CAD build for the part. Positions are in the model's coordinates, mm. Round coordinates to 2 decimals unless told otherwise and drop trailing zeros. Loops run counter-clockwise (first coordinate to the right, second up) from the corner with the lowest first, then second, coordinate; pieces in that order, holes last. Notation, with made-up numbers: M -0.5,20.25 L 42.5,20.25 A5 ccw 42.5,26.25 Z; hole C 84.25,-20.75 d1. An arc over 180 degrees is marked long. Use a Markdown table: item, result. Add a question column.
(1) Band-saw the part on D-D, the plane x = -10. Write the cut outline in (y, z), and give its area (3 significant figures).
(2) Band-saw the part on C-C, the plane z = 10. Write the cut outline in (x, y).
(3) Wall check: L1, parallel to Y at x = -0.5, z = -3; L2, parallel to X at y = -15, z = -7; L3, parallel to X at y = -15, z = 3. Give the ranges that are in metal, low to high.
(4) Flat gauge pins, fed straight in: P1, Ø8, axis at x = 0, y = -15, coming from the -Z side; P2, Ø8, axis at x = -8.5, y = -54.5, coming from the +Z side; P3, Ø2, axis at y = -100.5, z = 8.5, coming from the -X side; P4, Ø5, axis at y = -26.5, z = -9.5, coming from the +X side. Where does each tip first touch, or does it go through?
(5) Band-saw the part on B-B, the plane y = -125.5. Write the cut outline in (x, z), and give its area (3 significant figures).
(6) Band-saw the part on A-A, the plane z = -8.5. Write the cut outline in (x, y).
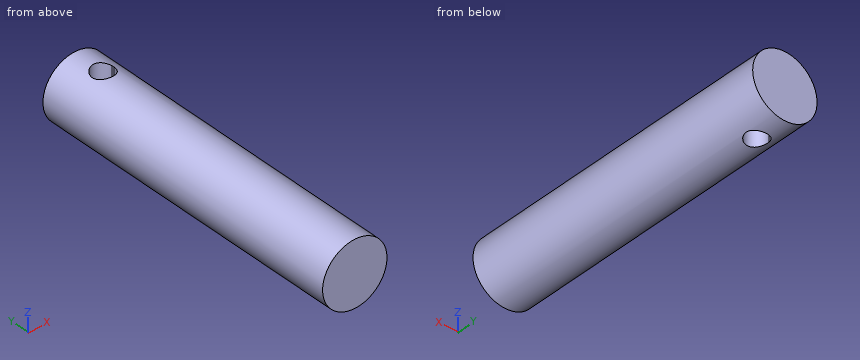
from build123d import *

# Parameters (mm, degrees)
F0_R     = 15
F1_DEPTH = 150
F3_DEPTH = 19.9


with BuildPart() as f1:
    # F0 (on Front) → F1 (new body)
    with BuildSketch(Plane.XZ):
        Circle(F0_R)
    extrude(amount=F1_DEPTH)

    # F2 (on Top) → F3 (cut, symmetric)
    with BuildSketch(Plane.XY):
        with BuildLine():
            ThreePointArc((4.9300664859, -14.1666666667), (0, -15), (-4.9300664859, -14.1666666667))
            ThreePointArc((-4.9300664859, -14.1666666667), (-0.4181313014, -19.9824859473), (5, -15))
            ThreePointArc((5, -15), (4.9824859473, -14.5818686986), (4.9300664859, -14.1666666667))
        make_face()
        with BuildLine():
            ThreePointArc((4.9300664859, -14.1666666667), (0, -10), (-4.9300664859, -14.1666666667))
            ThreePointArc((-4.9300664859, -14.1666666667), (0, -15), (4.9300664859, -14.1666666667))
        make_face()
    extrude(amount=F3_DEPTH, both=True, mode=Mode.SUBTRACT)


solid = f1.part
Return value:
| question | item | result |
|---|---|---|
| 1 | outline | M -150,-11.18 L 0,-11.18 L 0,11.18 L -150,11.18 Z |
| 1 | area | 3,350 mm^2 |
| 2 | outline | M -11.18,-150 L 11.18,-150 L 11.18,0 L -11.18,0 Z; hole C 0,-15 d10 |
| 3 | L1 | -150 to -19.97, -10.03 to 0 |
| 3 | L2 | -13.27 to -5, 5 to 13.27 |
| 3 | L3 | -14.7 to -5, 5 to 14.7 |
| 4 | P1 | through |
| 4 | P2 | z = 14.31 |
| 4 | P3 | x = -12.99 |
| 4 | P4 | x = 13.27 |
| 5 | outline | C 0,0 d30 |
| 5 | area | 707 mm^2 |
| 6 | outline | M -12.36,-150 L 12.36,-150 L 12.36,0 L -12.36,0 Z; hole C 0,-15 d10 |
